Build history of the part. All positions in model axes, mm. A direction names the side the tool comes from. Round coordinates to 2 decimals unless told otherwise and drop trailing zeros. Loops run counter-clockwise (first coordinate to the right, second up) from the corner with the lowest first, then second, coordinate; pieces in that order, holes last. Notation, with made-up numbers: M 42.25,-37 L 72.25,-37 A28 cw 72.25,-14 Z; hole C 60.25,78 d1. An arc over 180 degrees is marked long. One line per item, written item: value.
```python
from build123d import *

# Parameters (mm, degrees)
SKETCH1_R           = 4.05
SKETCH1_R_2         = 1.5
SKETCH1_R_3         = 2.004491684
SKETCH1_R_4         = 2.039529922
BOSS_EXTRUDE1_DEPTH = 10


with BuildPart() as part:
    # Sketch1 → Boss-Extrude1 (new body)
    with BuildSketch(Plane.XY):
        with BuildLine():
            Line((-36.50585994, 38), (23.49414006, 38))
            ThreePointArc((23.49414006, 38), (32.993428927, 36.45634395), (41.515142146, 31.984234067))
            Line((41.515142146, 31.984234067), (76.680353084, 5.562196244))
            ThreePointArc((76.680353084, 5.562196244), (79.334029485, -14.607546806), (59.473059994, -19.012365084))
            Line((59.473059994, -19.012365084), (33.489782569, -4.016722575))
            ThreePointArc((33.489782569, -4.016722575), (26.256281428, -1.021574208), (18.49414006, 0))
            Line((18.49414006, 0), (-31.50585994, 0))
            ThreePointArc((-31.50585994, 0), (-39.73032204, -1.149380887), (-47.324581503, -4.509451788))
            Line((-47.324581503, -4.509451788), (-102.315148598, -38.635060317))
            ThreePointArc((-102.315148598, -38.635060317), (-121.459805376, -36.232350563), (-123.106127076, -17.0078734))
            Line((-123.106127076, -17.0078734), (-53.947129798, 32.409057863))
            ThreePointArc((-53.947129798, 32.409057863), (-45.663596127, 36.56809178), (-36.50585994, 38))
        make_face()
        with Locations((66.99963225, -5.970908883)):
            Circle(SKETCH1_R, mode=Mode.SUBTRACT)
        with Locations((-44.575814379, 29.653127509)):
            Circle(SKETCH1_R_2, mode=Mode.SUBTRACT)
        with Locations((-115.847944697, -21.963472834)):
            Circle(SKETCH1_R_3, mode=Mode.SUBTRACT)
        with Locations((-109.381373154, -32.072055944)):
            Circle(SKETCH1_R_4, mode=Mode.SUBTRACT)
        with Locations(Location((-68.10465879, -5.666888812, 0), (0, 0, 180))):
            Circle(SKETCH1_R_4, mode=Mode.SUBTRACT)
        with Locations(Location((-74.571230332, 4.441694298, 0), (0, 0, 180))):
            Circle(SKETCH1_R_3, mode=Mode.SUBTRACT)
        with Locations((-40.818103787, 5.765583384)):
            Circle(SKETCH1_R_2, mode=Mode.SUBTRACT)
        with Locations((31.754938755, 29.566776323)):
            Circle(SKETCH1_R_2, mode=Mode.SUBTRACT)
        with Locations((27.4947716, 5.867993419)):
            Circle(SKETCH1_R_2, mode=Mode.SUBTRACT)
        Polygon((-114.633940841, -16.438421283), (-80.096281883, 5.655698153), (-69.318662645, -11.191940363), (-103.856321604, -33.286059799), align=None, mode=Mode.SUBTRACT)
        with BuildLine():
            Line((-23.016668441, 25.777290149), (11.250740888, 25.781094638))
            ThreePointArc((11.250740888, 25.781094638), (19.317386003, 17.716240499), (11.252531864, 9.649595384))
            Line((11.252531864, 9.649595384), (-23.014877464, 9.645790894))
            ThreePointArc((-23.014877464, 9.645790894), (-31.08152258, 17.710645033), (-23.016668441, 25.777290149))
        make_face(mode=Mode.SUBTRACT)
        with BuildLine():
            Line((39.069043687, 17.688629392), (55.302205937, 7.399981644))
            ThreePointArc((55.302205937, 7.399981644), (56.858473261, 0.45660111), (49.915092727, -1.099666214))
            Line((49.915092727, -1.099666214), (33.681930477, 9.188981534))
            ThreePointArc((33.681930477, 9.188981534), (32.125663153, 16.132362067), (39.069043687, 17.688629392))
        make_face(mode=Mode.SUBTRACT)
    extrude(amount=BOSS_EXTRUDE1_DEPTH)


solid = part.part
```
Item 1: Slice it at A-A, the plane y = -27. Give the cut face in (x, z).
Check values:
outline: M -125.68,0 L -107.88,0 L -107.88,10 L -125.68,10 Z; M -94.03,0 L -83.57,0 L -83.57,10 L -94.03,10 Z
Item 2: Pull direction Y, two halves, no side cores. Call faces 4 (the face through (-45.788, 36.528, 4.93)), 5 (the face through (-109.17, -24.98, 4.93)), 6 (the face through (-39.62, -1.12, 4.93)): pulls with the +Y half, pulls with the -Y half, needs draft (parallel to the pull), parting line crosses it, or undercut.
Check values:
face 4: pulls with the +Y half
face 5: undercut
face 6: pulls with the -Y half
Item 3: Slice it at B-B, the plane z = 7.25. Give the number of separate pieces and of enclosed holes in the cut face, and give its area (3 significant figures).
Check values:
separate pieces: 1
enclosed holes: 12
area: 5,580 mm2
Item 4: Slice it at C-C, the plane x = 68.5. Give the cut face in (y, z), and give its area (3 significant figures).
Check values:
outline: M -20.95,0 L -9.73,0 L -9.73,10 L -20.95,10 Z; M -2.21,0 L 11.71,0 L 11.71,10 L -2.21,10 Z
area: 251 mm2
Item 5: Which spindle directions (+Z, -Z, +X, -X, +Y, -Y) get a long thin tool onto all of the face, cutting with end or side? Do faces 1 (the face through (-6, 0, 5)), 2 (the face through (-7, 38, 5)), 3 (the face through (-97.61, -5.55, 4.93)). Say none if no direction does.
Check values:
face 1: +Z, -Z, -Y
face 2: +Z, -Z, +X, -X, +Y
face 3: +Z, -Z
Item 6: Wall check: line 1 along X through (y, z) = (-17.5, 5.5); line 2 along Y through (x, z) = (-108, 1.75); line 3 along X through (y, z) = (-8, 5.25). Give the ranges that are in metal, low to high.
Check values:
line 1: x = -123.43 to -113.95, -79.18 to -68.26, 56.85 to 76.69
line 2: y = -40.75 to -33.57, -30.57 to -26.81, -12.19 to -6.21
line 3: x = -110.5 to -101.44, -71.36 to -52.95, 40.39 to 63.49, 70.5 to 81.92
Item 7: Drop flat-ended pins along their axis: P1, Ø2, axis at y = 18.5, z = 6.5, coming from the +X side; P2, Ø3, axis at y = -18, z = 7, coming from the +X side; P3, Ø5, axis at x = -96, z = 3.5, coming from the -Y side. Give the stop position or say it passes through.
Check values:
P1: stops at x = 60.79
P2: stops at x = 77.76
P3: stops at y = -36.27
